CAD build for the part. Positions are in the model's coordinates, mm. A direction names the side the tool comes from. Round coordinates to 2 decimals unless told otherwise and drop trailing zeros. Write each loop counter-clockwise with the first axis right and the second up, starting at its lowest first coordinate (ties: lowest second). Pieces come first, ordered by that corner, then holes. Notation, with made-up numbers: (36.25, 13.5) - (50.25, 13.5) arc R11 cw to (50.25, 25.5) - close; hole circle Ø3 at (50, -27.75). An arc over 180 degrees is marked (long way). Put each result on its own line as item: value. Start each with the question number.
Item 1: Cut at B-B (z = 24.75). Give the cut face in (x, y), and give its area (4 significant figures).
Item 2: Mould opens along X. For faces 1 (the flat face through (-60.25, 2, 3)), 2 (the flat face through (-15, -2, 6.5)), 3 (the flat face through (27.5, -2, 17)), 4 (the flat face through (24, -2, 27)) say: released by +X, released by -X, zero draft, split by the parting line, or undercut.
Item 3: Cut at D-D (y = 13). Give the cut face in (x, z), and give its area (3 significant figures).
Item 4: Cut at C-C (z = 16.5). Give the cut face in (x, y), and give its area (4 significant figures).
Item 5: Drill centre lines: line 1 (X direction, y = -3.5, z = 21.75); line 2 (Z direction, x = -24, y = -6); line 3 (Y direction, x = -40.25, z = 0.65). Where is each one in solid material? Low to high. Write a range as from..to.
Item 6: Cut at A-A (x = -40.25). Give the cut face in (y, z), and give its area (3 significant figures).
Item 7: 3-axis set-ups, long thin cutter, end or side, ignore diameter. For faces 5 (the flat face through (-27.5, -2, 17)), 6 (the flat face through (-20.25, -2, 17)), 7 (the cylindrical face through (-50.74, 14.71, 3.94)), 8 (the flat face through (24, 6.5, 17)), 9 (the flat face through (0, 16.5, 17)): which of +Z, -Z, +X, -X, +Y, -Y reach the whole face in a straight line?
Item 8: Pin check, flat tips, straight feed: pin 1 Ø2 at (x, z) = (25, 18.5) entering from -Y; pin 2 Ø12.5 at (x, y) = (-40.25, 14.25) entering from +Z; pin 3 Ø8 at (y, z) = (-10, 14) entering from -X. Stop position of each tip, or through.
```python
from build123d import *

# Parameters (mm, degrees)
ESQUISSE1_W              = 55
ESQUISSE1_H              = 43
BOSS_EXTRU_1_DEPTH       = 27
ESQUISSE2_W              = 40.5
ESQUISSE2_H              = 21.676575317
ENL_V_MAT_EXTRU_1_DEPTH  = 38
ESQUISSE3_R              = 0.7
ENL_V_MAT_EXTRU_2_DEPTH  = 43
ESQUISSE4_W              = 55
ESQUISSE4_H              = 20.5
ENL_V_MAT_EXTRU_3_DEPTH  = 11
ENL_V_MAT_EXTRU_6_REACH  = 66.933
ESQUISSE5_W              = 20.5
ESQUISSE5_H              = 10
ESQUISSE6_W              = 7.25
ESQUISSE6_H              = 20.5
ENL_V_MAT_EXTRU_7_DEPTH  = 5
ESQUISSE7_R              = 31
BOSS_EXTRU_2_DEPTH       = 6.5
ESQUISSE8_R              = 41
ESQUISSE8_R_2            = 31
ENL_V_MAT_EXTRU_8_DEPTH  = 6.5
TROU_TARAUD_M2X0_41_D    = 1.6
ESQUISSE10_R             = 10.5
ENL_V_MAT_EXTRU_9_DEPTH  = 4.5
ESQUISSE11_R             = 4.5
ENL_V_MAT_EXTRU_10_DEPTH = 2
ESQUISSE12_R             = 9.25
ESQUISSE12_R_2           = 1.25
BOSS_EXTRU_3_DEPTH       = 5
ESQUISSE13_W             = 50.114904395
ESQUISSE13_H             = 12.012600019
ENL_V_MAT_EXTRU_11_DEPTH = 6.5
BOSS_EXTRU_4_START       = 1.2
BOSS_EXTRU_4_DEPTH       = 1.2
ESQUISSE15_W             = 53.005482756
ESQUISSE15_H             = 10
ENL_V_MAT_EXTRU_12_DEPTH = 7.7
ESQUISSE16_R             = 4.5
ENL_V_MAT_EXTRU_13_DEPTH = 1.2
BOSS_EXTRU_5_START       = -28.2
ESQUISSE17_W             = 40.5
ESQUISSE17_H             = 5
BOSS_EXTRU_5_DEPTH       = 28.2
ESQUISSE18_R             = 1
ENL_V_MAT_EXTRU_14_DEPTH = 10
TROU_TARAUD_M3X0_51_D    = 2.5
ESQUISSE22_R             = 4.5
BOSS_EXTRU_6_DEPTH       = 7.7
ESQUISSE23_R             = 10.5
ENL_V_MAT_EXTRU_15_DEPTH = 5.2
ESQUISSE24_R             = 12.885190895
BOSS_EXTRU_7_DEPTH       = 7.7


with BuildPart() as part:
    # Esquisse1 → Boss.-Extru.1 (new body)
    with BuildSketch(Plane.XY):
        Rectangle(ESQUISSE1_W, ESQUISSE1_H)
    extrude(amount=BOSS_EXTRU_1_DEPTH)

    # Esquisse2 → Enlèv. mat.-Extru.1 (cut)
    with BuildSketch(Plane.XZ.offset(21.5)):
        with Locations((0, 17.338287659)):
            Rectangle(ESQUISSE2_W, ESQUISSE2_H)
    extrude(amount=-ENL_V_MAT_EXTRU_1_DEPTH, mode=Mode.SUBTRACT)

    # Esquisse3 → Enlèv. mat.-Extru.2 (cut)
    with BuildSketch(Plane.XZ.offset(21.5)):
        with Locations(Location((-24.71, 21.675, 0), (0, 0, 270))):
            Circle(ESQUISSE3_R)
        with Locations(Location((-24.71, 11.825, 0), (0, 0, 270))):
            Circle(ESQUISSE3_R)
        with Locations(Location((24.71, 11.825, 0), (0, 0, 270))):
            Circle(ESQUISSE3_R)
        with Locations(Location((24.71, 21.675, 0), (0, 0, 270))):
            Circle(ESQUISSE3_R)
    extrude(amount=-ENL_V_MAT_EXTRU_2_DEPTH, mode=Mode.SUBTRACT)

    # Esquisse4 → Enlèv. mat.-Extru.3 (cut)
    with BuildSketch(Plane.XZ.offset(21.5)):
        with Locations((0, 16.75)):
            Rectangle(ESQUISSE4_W, ESQUISSE4_H)
    extrude(amount=-ENL_V_MAT_EXTRU_3_DEPTH, mode=Mode.SUBTRACT)

    # Enlèv. mat.-Extru.6: up to this face of the body (flat: up to its plane)
    enl_v_mat_extru_6_end = Plane(part.part.faces().sort_by_distance((27.5, 3.85676109, 12.716595404))[0])
    # Esquisse5 → Enlèv. mat.-Extru.6 (cut, up to the picked face)
    with BuildSketch(Plane.ZY.offset(27.5), mode=Mode.PRIVATE) as enl_v_mat_extru_6_sk1:
        with Locations((16.75, 11.5)):
            Rectangle(ESQUISSE5_W, ESQUISSE5_H)
    enl_v_mat_extru_6_tool1 = split(extrude(enl_v_mat_extru_6_sk1.sketch, amount=-ENL_V_MAT_EXTRU_6_REACH, mode=Mode.PRIVATE), bisect_by=enl_v_mat_extru_6_end, keep=Keep.BOTH, mode=Mode.PRIVATE)
    add(enl_v_mat_extru_6_tool1.solids().sort_by(Axis((-27.5, 11.5, 16.75), (1, 0, 0)))[0], mode=Mode.SUBTRACT)

    # Esquisse6 → Enlèv. mat.-Extru.7 (cut)
    with BuildSketch(Plane.XZ.offset(-16.5)):
        with Locations((-23.875, 16.75)):
            Rectangle(ESQUISSE6_W, ESQUISSE6_H)
        with Locations((23.875, 16.75)):
            Rectangle(ESQUISSE6_W, ESQUISSE6_H)
    extrude(amount=-ENL_V_MAT_EXTRU_7_DEPTH, mode=Mode.SUBTRACT)

    # Esquisse7 → Boss.-Extru.2 (add)
    with BuildSketch(Plane(origin=(0, 0, 0), x_dir=(-1, 0, 0), z_dir=(0, 0, -1))):
        Circle(ESQUISSE7_R)
    extrude(amount=-BOSS_EXTRU_2_DEPTH)

    # Esquisse8 → Enlèv. mat.-Extru.8 (cut)
    with BuildSketch(Plane(origin=(0, 0, 0), x_dir=(-1, 0, 0), z_dir=(0, 0, -1))):
        Circle(ESQUISSE8_R)
        Circle(ESQUISSE8_R_2, mode=Mode.SUBTRACT)
    extrude(amount=-ENL_V_MAT_EXTRU_8_DEPTH, mode=Mode.SUBTRACT)

    # Trou taraudé M2x0.41 (through all)
    with Locations(Plane(origin=(-24.71, -10.5, 21.675), x_dir=(0, 0, -1), z_dir=(0, -1, 0))):
        with Locations((0, 0), (9.85, 0), (0, 49.42), (9.85, 49.42)):
            Hole(TROU_TARAUD_M2X0_41_D / 2)

    # Esquisse10 → Enlèv. mat.-Extru.9 (cut)
    with BuildSketch(Plane.XY.offset(6.5)):
        Circle(ESQUISSE10_R)
    extrude(amount=-ENL_V_MAT_EXTRU_9_DEPTH, mode=Mode.SUBTRACT)

    # Esquisse11 → Enlèv. mat.-Extru.10 (cut)
    with BuildSketch(Plane.XY.offset(2)):
        Circle(ESQUISSE11_R)
    extrude(amount=-ENL_V_MAT_EXTRU_10_DEPTH, mode=Mode.SUBTRACT)

    # Esquisse12 → Boss.-Extru.3 (add)
    with BuildSketch(Plane(origin=(0, 21.5, 0), x_dir=(1, 0, 0), z_dir=(0, 1, 0))):
        with Locations(Location((0, -15.876822983, 0), (0, 0, 90))):
            Circle(ESQUISSE12_R)
        with Locations(Location((0, -15.876822983, 0), (0, 0, 270))):
            Circle(ESQUISSE12_R_2, mode=Mode.SUBTRACT)
    extrude(amount=BOSS_EXTRU_3_DEPTH)

    # Esquisse13 → Enlèv. mat.-Extru.11 (cut)
    with BuildSketch(Plane.XY.offset(6.5)):
        with Locations((-0.983340997, 27.50630001)):
            Rectangle(ESQUISSE13_W, ESQUISSE13_H)
    extrude(amount=-ENL_V_MAT_EXTRU_11_DEPTH, mode=Mode.SUBTRACT)

    # Esquisse14 → Boss.-Extru.4 (add)
    with BuildSketch(Plane(origin=(0, 0, 0), x_dir=(-1, 0, 0), z_dir=(0, 0, -1)).offset(BOSS_EXTRU_4_START)):
        with BuildLine():
            Line((-22.332711434, 21.5), (22.332711434, 21.5))
            ThreePointArc((22.332711434, 21.5), (0, -31), (-22.332711434, 21.5))
        make_face()
    extrude(amount=-BOSS_EXTRU_4_DEPTH)

    # Esquisse15 → Enlèv. mat.-Extru.12 (cut)
    with BuildSketch(Plane.XY.offset(6.5)):
        with Locations((0, -26)):
            Rectangle(ESQUISSE15_W, ESQUISSE15_H)
    extrude(amount=-ENL_V_MAT_EXTRU_12_DEPTH, mode=Mode.SUBTRACT)

    # Esquisse16 → Enlèv. mat.-Extru.13 (cut)
    with BuildSketch(Plane.XY):
        Circle(ESQUISSE16_R)
    extrude(amount=-ENL_V_MAT_EXTRU_13_DEPTH, mode=Mode.SUBTRACT)

    # Esquisse17 → Boss.-Extru.5 (add)
    with BuildSketch(Plane.XY.offset(27).offset(BOSS_EXTRU_5_START)):
        with Locations((0, 24)):
            Rectangle(ESQUISSE17_W, ESQUISSE17_H)
    extrude(amount=BOSS_EXTRU_5_DEPTH)

    # Esquisse18 → Enlèv. mat.-Extru.14 (cut)
    with BuildSketch(Plane(origin=(0, 26.5, 0), x_dir=(1, 0, 0), z_dir=(0, 1, 0))):
        with Locations(Location((9.65, -16.5, 0), (0, 0, 270))):
            Circle(ESQUISSE18_R)
    extrude(amount=-ENL_V_MAT_EXTRU_14_DEPTH, mode=Mode.SUBTRACT)

    # Trou taraudé M3x0.51 (through all)
    with Locations(Plane(origin=(9.65, 26.5, 16.5), x_dir=(0, 0, 1), z_dir=(0, 1, 0))):
        with Locations((0, 0)):
            Hole(TROU_TARAUD_M3X0_51_D / 2)

    # Esquisse22 → Boss.-Extru.6 (add)
    with BuildSketch(Plane(origin=(0, 0, -1.2), x_dir=(-1, 0, 0), z_dir=(0, 0, -1))):
        Polygon((20.25, 26.5), (60.25, 26.5), (60.25, 2), (60.25, -21), (20.25, -21), (20.25, 2), align=None)
        with Locations((40.25, 14.25)):
            Circle(ESQUISSE22_R, mode=Mode.SUBTRACT)
    extrude(amount=-BOSS_EXTRU_6_DEPTH)

    # Esquisse23 → Enlèv. mat.-Extru.15 (cut)
    with BuildSketch(Plane.XY.offset(6.5)):
        with Locations((-40.25, 14.25)):
            Circle(ESQUISSE23_R)
    extrude(amount=-ENL_V_MAT_EXTRU_15_DEPTH, mode=Mode.SUBTRACT)

    # Esquisse24 → Boss.-Extru.7 (add)
    with BuildSketch(Plane(origin=(0, 0, -1.2), x_dir=(-1, 0, 0), z_dir=(0, 0, -1))):
        Circle(ESQUISSE24_R)
    extrude(amount=-BOSS_EXTRU_7_DEPTH)


solid = part.part
```
Output values:
1. outline: (-27.5, -10.5) - (-20.25, -10.5) - (-20.25, 6.5) - (-27.5, 6.5) - close; (-20.25, 16.5) - (20.25, 16.5) - (20.25, 26.5) - (-20.25, 26.5) - close; (20.25, -10.5) - (27.5, -10.5) - (27.5, 6.5) - (20.25, 6.5) - close
1. area: 651.5 mm2
2. face 1: released by -X
2. face 2: undercut
2. face 3: released by +X
2. face 4: zero draft
3. outline: (-60.25, -1.2) - (-44.57, -1.2) - (-44.57, 1.3) - (-50.68, 1.3) - (-50.68, 6.5) - (-60.25, 6.5) - close; (-35.93, -1.2) - (28.14, -1.2) - (28.14, 6.5) - (-29.82, 6.5) - (-29.82, 1.3) - (-35.93, 1.3) - close
3. area: 551 mm2
4. outline: (-27.5, -10.5) - (-20.25, -10.5) - (-20.25, 6.5) - (-27.5, 6.5) - close; (-20.25, 16.5) - (8.4, 16.5) - (8.4, 26.5) - (-20.25, 26.5) - close; (10.9, 16.5) - (20.25, 16.5) - (20.25, 26.5) - (10.9, 26.5) - close; (20.25, -10.5) - (27.5, -10.5) - (27.5, 6.5) - (20.25, 6.5) - close
4. area: 626.5 mm2
5. line 1: -27.5..-25.51, -23.91..-20.25, 20.25..23.91, 25.51..27.5
5. line 2: -1.2..11.46, 12.19..21.31, 22.04..27
5. line 3: -21..9.75, 18.75..26.5
6. outline: (-21, -1.2) - (9.75, -1.2) - (9.75, 1.3) - (3.75, 1.3) - (3.75, 6.5) - (-21, 6.5) - close; (18.75, -1.2) - (26.5, -1.2) - (26.5, 6.5) - (24.75, 6.5) - (24.75, 1.3) - (18.75, 1.3) - close
6. area: 234 mm2
7. face 5: +Z, -X, +Y, -Y
7. face 6: +Z, -Y
7. face 7: +Z
7. face 8: +Z, +X, -X, +Y
7. face 9: +Z, +X, -X, -Y
8. pin 1: y = -10.5
8. pin 2: z = 1.3
8. pin 3: x = -27.5
